CAD build for the part. Positions are in the model's coordinates, mm. A direction names the side the tool comes from. Give positions to 0.01 mm unless a question says otherwise; leave off trailing zeros. Order: outer loops, then holes, each group sorted by start corner. A loop starts at its lowest first (then second) coordinate and runs counter-clockwise, first axis right, second up.
from build123d import *

# Parameters (mm, degrees)
IZIM1_W                     = 30
IZIM1_H                     = 30
Y_KSEKLIK_EKSTR_ZYON1_DEPTH = 6
IZIM2_W                     = 30
IZIM2_H                     = 6
KES_EKSTR_ZYON1_DEPTH       = 4
IZIM3_W                     = 30
IZIM3_H                     = 6
KES_EKSTR_ZYON2_DEPTH       = 4
IZIM4_R                     = 9
Y_KSEKLIK_EKSTR_ZYON2_DEPTH = 19.5
IZIM5_R                     = 6
Y_KSEKLIK_EKSTR_ZYON3_DEPTH = 24


with BuildPart() as part:
    # Çizim1 → Yükseklik-Ekstrüzyon1 (new body)
    with BuildSketch(Plane.XY):
        with Locations((-24.193211068, 8.69047619)):
            Rectangle(IZIM1_W, IZIM1_H)
    extrude(amount=Y_KSEKLIK_EKSTR_ZYON1_DEPTH)

    # Çizim2 → Kes-Ekstrüzyon1 (cut)
    with BuildSketch(Plane.XY.offset(6)):
        with Locations((-24.193211068, -3.30952381)):
            Rectangle(IZIM2_W, IZIM2_H)
    extrude(amount=-KES_EKSTR_ZYON1_DEPTH, mode=Mode.SUBTRACT)

    # Çizim3 → Kes-Ekstrüzyon2 (cut)
    with BuildSketch(Plane.XY.offset(6)):
        with Locations((-24.193211068, 20.69047619)):
            Rectangle(IZIM3_W, IZIM3_H)
    extrude(amount=-KES_EKSTR_ZYON2_DEPTH, mode=Mode.SUBTRACT)

    # Çizim4 → Yükseklik-Ekstrüzyon2 (add)
    with BuildSketch(Plane(origin=(0, 0, 0), x_dir=(-1, 0, 0), z_dir=(0, 0, -1))):
        with Locations((24.193211068, 8.69047619)):
            Circle(IZIM4_R)
    extrude(amount=Y_KSEKLIK_EKSTR_ZYON2_DEPTH)

    # Çizim5 → Yükseklik-Ekstrüzyon3 (add)
    with BuildSketch(Plane(origin=(0, 0, -19.5), x_dir=(-1, 0, 0), z_dir=(0, 0, -1))):
        with Locations((24.193211068, 8.69047619)):
            Circle(IZIM5_R)
    extrude(amount=Y_KSEKLIK_EKSTR_ZYON3_DEPTH)


solid = part.part
1. Saw through at A-A on x = -12.25. Give the cut face in (y, z).
2. 3-axis set-ups, long thin cutter, end or side, ignore diameter. For faces 1 (the cylindrical face through (-28.35, 0.71, -9.61)), 2 (the flat face through (-24, 21, 2)), 3 (the flat face through (-24, -0.31, 4)): which of +Z, -Z, +X, -X, +Y, -Y reach the whole face in a straight line?
3. Saw through at D-D on y = 17. Give the cut face in (x, z).
4. Saw through at C-C on z = -14.5. Give the cut face in (x, y).
5. Pin check, flat tips, straight feed: P1, Ø8, axis at y = 6, z = -21.5, coming from the +X side; P2, Ø1, axis at x = -24.5, z = -2, coming from the -Y side; P3, Ø3, axis at y = 14.5, z = -37, coming from the +X side; P4, Ø5, axis at y = -1, z = -23, coming from the +X side. Stop position of each tip, or through.
6. Saw through at B-B on y = 6.25. Give the cut face in (x, z), plus the area to 3 significant figures.
7. Wall check: line 1 (Z direction, x = -36.75, y = 1.5); line 2 (Z direction, x = -17.25, y = 21.75); line 3 (Y direction, x = -20.5, z = -33.5). Give the ranges that are in metal, low to high.
Reported:
1. outline: (-6.31, 0) - (23.69, 0) - (23.69, 2) - (17.69, 2) - (17.69, 6) - (-0.31, 6) - (-0.31, 2) - (-6.31, 2) - close
2. face 1: -Z
2. face 2: +Z, +X, -X, +Y
2. face 3: +Z, +X, -X, -Y
3. outline: (-39.19, 0) - (-27.65, 0) - (-27.65, -19.5) - (-20.74, -19.5) - (-20.74, 0) - (-9.19, 0) - (-9.19, 6) - (-39.19, 6) - close
4. outline: circle Ø18 at (-24.19, 8.69)
5. P1: stops at x = -15.19
5. P2: stops at y = -0.31
5. P3: stops at x = -20.02
5. P4: passes through
6. outline: (-39.19, 0) - (-32.86, 0) - (-32.86, -19.5) - (-29.67, -19.5) - (-29.67, -43.5) - (-18.71, -43.5) - (-18.71, -19.5) - (-15.53, -19.5) - (-15.53, 0) - (-9.19, 0) - (-9.19, 6) - (-39.19, 6) - close
6. area: 781 mm2
7. line 1: z = 0 to 6
7. line 2: z = 0 to 2
7. line 3: y = 3.96 to 13.42
